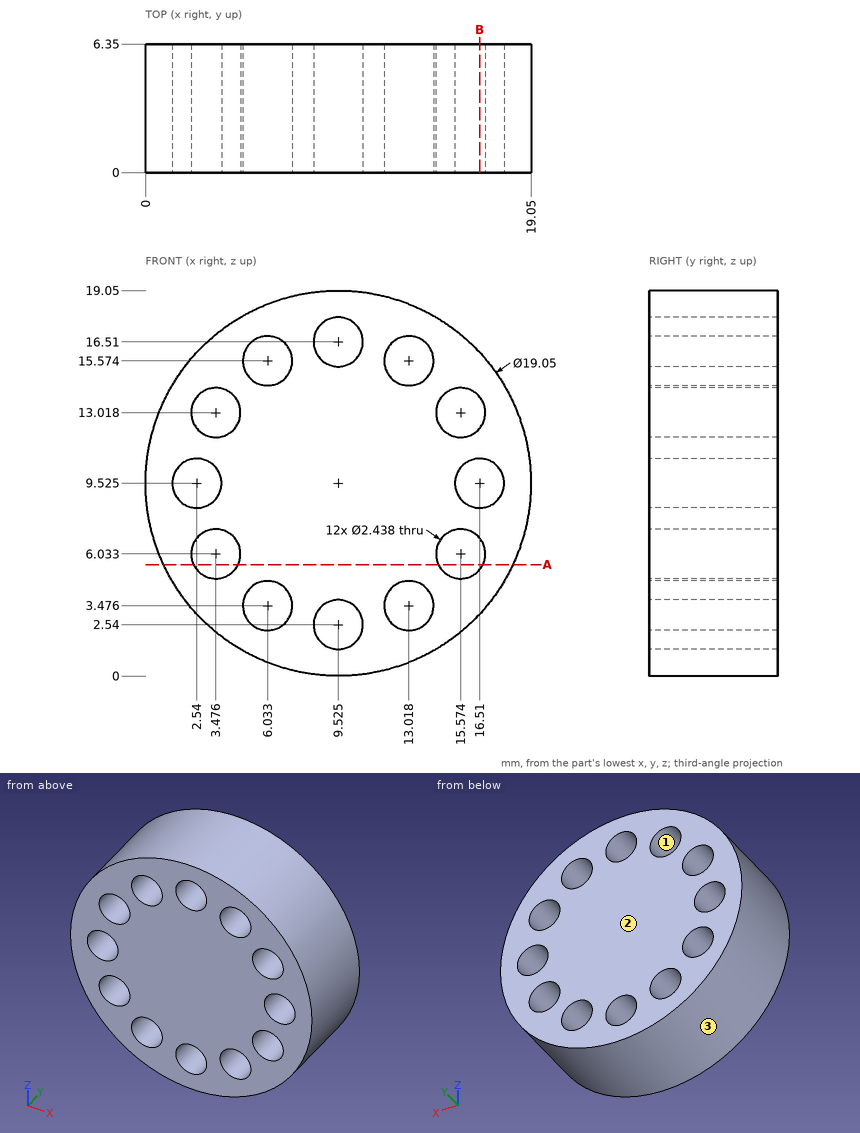
The drawing under review shows one solid part. Ordinate dimensions are in mm from its lowest x, y, z. Round coordinates to 2 decimals unless told otherwise and drop trailing zeros. Write each loop counter-clockwise with the first axis right and the second up, starting at its lowest first coordinate (ties: lowest second). Pieces come first, ordered by that corner, then holes. Notation, with made-up numbers: M 26,-7.5 L 73,-7.5 A23 ccw 73,18.5 Z; hole C 34,75 d7. An arc over 180 degrees is marked long. One line per item, written item: value. Start each with the question number.
(1) Wall thickness on line 1 (X direction, y = 1.5, z = 6) (1 decimal); line 2 (Z direction, x = 9.25, y = 2) (1 decimal); line 3 (Z direction, x = 1.25, y = 1.25) (1 decimal): over which ranges is each line inside the solid? List them lowest first.
(2) Insertion check: pin 1 (3 mm diameter, centred on y = 1, z = 7.5, fed in from -X) (1 decimal); pin 2 (2 mm diameter, centred on x = 13, y = 2, fed in from +Z); pin 3 (1.5 mm diameter, centred on y = 1.5, z = 5, fed in from +X). Each pin has a flat end and moves straight along its axis. Give the tip position at first contact, or say it passes through.
(3) We need section B-B (x = 16.51). Count the separate pieces of the cut face and the enclosed holes in it.
(4) The part is to be moulded in two halves that separate along Z. For the marked faces 1, 2 and 3, say which applies: released by +Z, released by -Z, zero draft, split by the parting line, or undercut.
(5) We need section A-A (z = 5.5). Give the boundary of the cut face in (x, y).
Result:
1. line 1: 0.7 to 2.3, 4.7 to 14.4, 16.8 to 18.4
1. line 2: 0 to 1.4, 3.7 to 15.3, 17.7 to 19
1. line 3: 4.8 to 14.2
2. pin 1: x = 0
2. pin 2: z = 18.72
2. pin 3: x = 18.27
3. separate pieces: 4
3. enclosed holes: 0
4. face 1: undercut
4. face 2: zero draft
4. face 3: split by the parting line
5. outline: M 0.89,0 L 2.38,0 L 2.38,6.35 L 0.89,6.35 Z; M 4.57,0 L 14.48,0 L 14.48,6.35 L 4.57,6.35 Z; M 16.67,0 L 18.16,0 L 18.16,6.35 L 16.67,6.35 Z
